Input: dimensioned drawing with shaded views. Units: mm. Origin: part minimum x, y, z. A direction names the side the tool comes from. Round coordinates to 2 decimals unless told otherwise and drop trailing zeros. Loops run counter-clockwise (first coordinate to the right, second up) from the corner with the lowest first, then second, coordinate; pieces in that order, holes last. Notation, with made-up numbers: (77.5, -36) - (81.5, -36) arc R17 ccw to (81.5, -17) - close; hole circle Ø10 at (16, -24). An arc over 180 degrees is marked (long way). One line per question, with ' | ' between items. Start each with the question number.
1. Cut plane A-A (y = 14). Return loops of the section in (x, z).
2. Pin query (flat end, axial travel): pin 1 (10 mm diameter, centred on x = 11, y = 12, fed in from +Z); pin 2 (1.5 mm diameter, centred on x = 20, z = 36, fed in from +Y); pin 3 (4 mm diameter, centred on y = 6, z = 19.5, fed in from -X). Return the tip coordinate at first contact, or that it passes through.
3. Ray query, line 1 (Z direction, x = 27, y = 25); line 2 (Z direction, x = 20.5, y = 23); line 3 (Y direction, x = 21, z = 34). Return the intervals inside material, ascending.
4. Cut plane D-D (z = 58). Return loops of the section in (x, y), then the cut area to 3 significant figures.
5. Access query for the marked faces 1 and 2. Directions: +Z, -Z, +X, -X, +Y, -Y. A direction counts if a zero-diameter tool reaches every point of the face in a straight line with its end or side. Return the directions, or none.
6. Cut plane C-C (x = 21.5). Return loops of the section in (y, z), then the cut area to 3 significant figures.
7. Cut plane B-B (z = 8.5). Return loops of the section in (x, y).
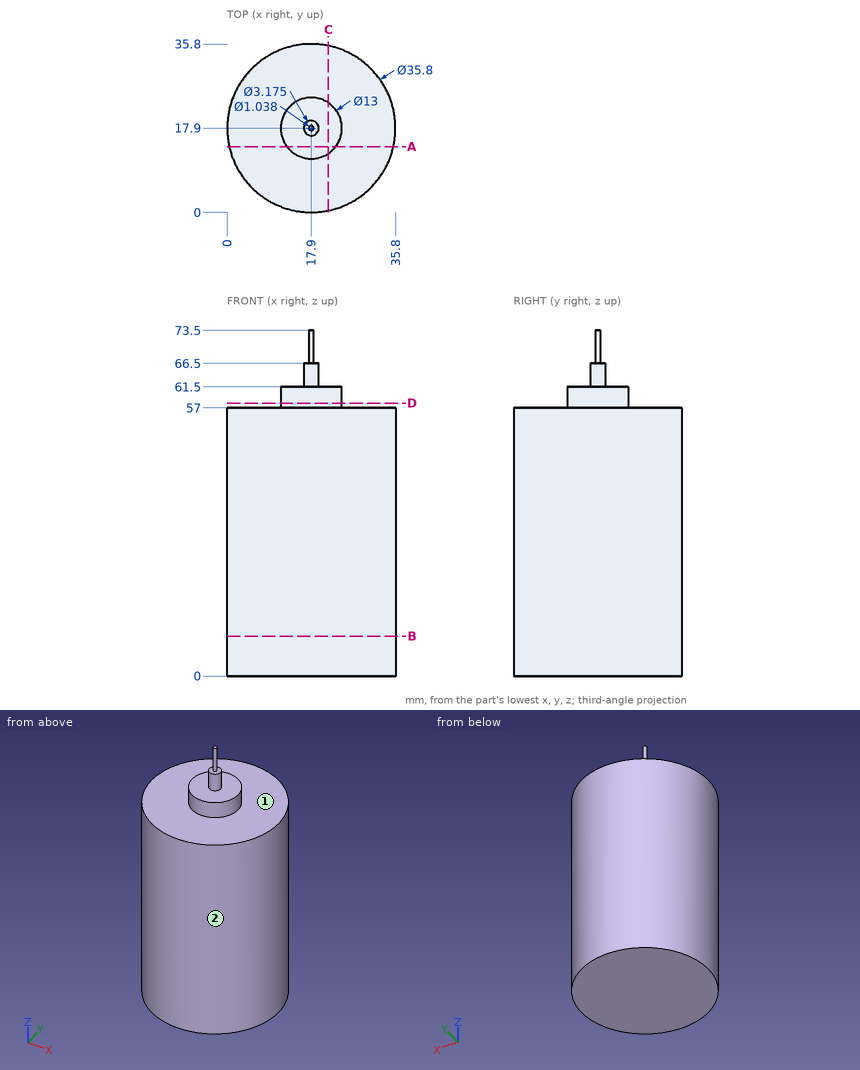
Answers follow:
1) outline: (0.43, 0) - (35.37, 0) - (35.37, 57) - (23.1, 57) - (23.1, 61.5) - (12.7, 61.5) - (12.7, 57) - (0.43, 57) - close
2) pin 1: stops at z = 61.5 | pin 2: stops at y = 35.75 | pin 3: stops at x = 2.99
3) line 1: z = 0 to 57 | line 2: z = 0 to 61.5 | line 3: y = 0.27 to 35.53
4) outline: circle Ø13 at (17.9, 17.9) | area: 133 mm2
5) face 1: +Z | face 2: +Z, -Z
6) outline: (0.37, 0) - (35.43, 0) - (35.43, 57) - (23.31, 57) - (23.31, 61.5) - (12.49, 61.5) - (12.49, 57) - (0.37, 57) - close | area: 2,050 mm2
7) outline: circle Ø35.8 at (17.9, 17.9)
